Autodesk Inventor part; units mm, degrees
ref_plane "YZ Plane" through (0, 0, 0) normal (1, 0, 0) x (0, 1, 0)
ref_plane "XZ Plane" through (0, 0, 0) normal (0, 1, 0) x (-1, 0, 0)
ref_plane "XY Plane" through (0, 0, 0) normal (0, 0, 1) x (1, 0, 0)
sketch "Sketch1" plane through (0, 0, 0) normal (0, 1, 0) x (-1, 0, 0)
  line L0 (140, 140) -> (-140, 140)
  line L1 (-140, 140) -> (-140, -140)
  line L2 (-140, -140) -> (140, -140)
  line L3 (140, -140) -> (140, 140)
  point P0 (0, 0)
  point P1 (140, 0)
  point P2 (0, -140)
  dimension "d0" = 280
  dimension "d1" = 280
extrude "Extrusion1" add sketch "Sketch1" along normal blind 10
sketch "Sketch2" plane through (0, 10, 0) normal (0, 1, 0) x (1, 0, 0)
  line L0 (-140, -140) -> (140, -140)
  line L1 (140, -140) -> (140, 140)
  line L2 (140, 140) -> (-140, 140)
  line L3 (-140, 140) -> (-140, -140)
  line L4 (-132, -132) -> (132, -132)
  line L5 (132, -132) -> (132, 132)
  line L6 (132, 132) -> (-132, 132)
  line L7 (-132, 132) -> (-132, -132)
  point P0 (0, 0)
  dimension "d4" = 8
extrude "Extrusion2" add sketch "Sketch2" along normal blind 150
sketch "Sketch3" plane through (0, 160, 0) normal (0, 1, 0) x (1, 0, 0)
  circle A0 centre (-135, 135) radius 2.05
  circle A1 centre (135, 135) radius 2.05
  circle A2 centre (135, -135) radius 2.05
  circle A3 centre (-135, -135) radius 2.05
  line L0 (140, -140) -> (140, 140)
  line L1 (-140, -140) -> (140, -140)
  line L2 (140, 140) -> (-140, 140)
  line L3 (-140, 140) -> (-140, -140)
  point P0 (0, 0)
  dimension "d8" = 4.1
  dimension "d12" = 5
  dimension "d16" = 5
  dimension "d18" = 4.1
  dimension "d19" = 5
  dimension "d20" = 5
  dimension "d21" = 4.1
  dimension "d22" = 5
  dimension "d23" = 5
  dimension "d24" = 5
  dimension "d25" = 5
  dimension "d26" = 4.1
extrude "Extrusion3" cut sketch "Sketch3" against normal blind 15 contours A0 | A1 | A2 | A3
sketch "Sketch4" plane through (140, 0, 140) normal (1, 0, 0) x (0, 0, -1)
  line L0 (90, 130) -> (190, 130)
  line L1 (190, 130) -> (190, 30)
  line L2 (190, 30) -> (90, 30)
  line L3 (90, 30) -> (90, 130)
  line L4 (0, 160) -> (280, 160)
  line L5 (280, 0) -> (280, 160)
  point P0 (140, 0)
  point P1 (140, 130)
  point P2 (140, 160)
  point P3 (190, 80)
  point P4 (280, 80)
  dimension "d29" = 100
  dimension "d30" = 100
sketch "Sketch5" plane through (-140, 0, 140) normal (0, 0, 1) x (1, 0, 0)
  line L0 (280, 0) -> (280, 160)
  line L1 (0, 160) -> (280, 160)
  circle A0 centre (140, 80) radius 40.5
  point P0 (140, 0)
  point P1 (195.958, 80)
  point P2 (280, 80)
  point P3 (140, 107.0458)
  point P4 (140, 160)
  point P5 (280, 80)
  point P6 (140, 160)
  dimension "d81" = 81
extrude "Extrusion4" cut sketch "Sketch5" against normal blind 10
sketch "Sketch6" plane through (-140, 0, 140) normal (0, 0, 1) x (1, 0, 0)
  line L0 (192.5, 27.5) -> (87.5, 27.5)
  line L1 (87.5, 27.5) -> (87.5, 132.5)
  line L2 (87.5, 132.5) -> (192.5, 132.5)
  line L3 (192.5, 132.5) -> (192.5, 27.5)
  line L4 (0, 0) -> (280, 0)
  line L5 (0, 0) -> (0, 160)
  circle A0 centre (182.5, 37.5) radius 2.75
  circle A1 centre (182.5, 122.5) radius 2.75
  circle A2 centre (97.5, 37.5) radius 2.75
  circle A3 centre (97.5, 122.5) radius 2.75
  line L6 (210, 30) -> (70, 30)
  point P0 (140, 0)
  point P1 (49.5, 158)
  point P2 (180.5, 27)
  point P3 (140, 27.5)
  point P4 (140, 0)
  point P5 (87.5, 80)
  point P6 (0, 80)
  point P7 (60, 80)
  point P8 (140, 30)
  dimension "d108" = 105
  dimension "d109" = 105
  dimension "d112" = 5.5
  dimension "d113" = 10
  dimension "d114" = 10
  dimension "d117" = 85
  dimension "d120" = 85
sketch "Sketch7" plane through (0, 10, 0) normal (0, 1, 0) x (1, 0, 0)
  line L0 (132, 132) -> (132, -132) construction
  line L1 (132, 0) -> (-132, 0) construction
  line L2 (-132, -132) -> (-132, 132) construction
  point P0 (0, 0)
ref_plane "Work Plane1" through (132, 10, 0) normal (0, 0, -1) x (-1, 0, 0)
extrude "Extrusion13" cut sketch "Sketch6" against normal blind 5
mirror "Mirror2" about plane through (132, 10, 0) normal (0, 0, -1) of "Extrusion4"
sketch "Sketch8" plane through (0, 0, 0) normal (0, -1, 0) x (1, 0, 0)
  line L0 (75, -75) -> (-75, -75)
  line L1 (-75, -75) -> (-75, 75)
  line L2 (-75, 75) -> (75, 75)
  line L3 (75, 75) -> (75, -75)
  circle A0 centre (65, -65) radius 2.75
  circle A1 centre (65, 65) radius 2.75
  circle A2 centre (-65, -65) radius 2.75
  circle A3 centre (-65, 65) radius 2.75
  circle A4 centre (0, 0) radius 40.5
  point P0 (-35, 0)
  point P1 (0, -35)
  point P2 (75, 0)
  point P3 (0, -75)
  dimension "d58" = 130
  dimension "d65" = 130
  dimension "d82" = 81
  dimension "d83" = 150
  dimension "d84" = 150
  dimension "d85" = 10
  dimension "d86" = 10
  dimension "d87" = 130
  dimension "d88" = 130
  dimension "d89" = 5.5
  dimension "d90" = 5.5
  dimension "d91" = 5.5
  dimension "d92" = 5.5
extrude "Extrusion9" cut sketch "Sketch8" against normal blind 10 contours A4
sketch "Sketch13" plane through (0, 0, 0) normal (0, -1, 0) x (1, 0, 0)
  line L0 (-52.5, 52.5) -> (52.5, 52.5)
  line L1 (52.5, 52.5) -> (52.5, -52.5)
  line L2 (52.5, -52.5) -> (-52.5, -52.5)
  line L3 (-52.5, -52.5) -> (-52.5, 52.5)
  circle A0 centre (-42.5, 42.5) radius 2.75
  circle A1 centre (-42.5, -42.5) radius 2.75
  circle A2 centre (42.5, -42.5) radius 2.75
  circle A3 centre (42.5, 42.5) radius 2.75
  point P0 (0, 0)
  point P1 (52.5, 0)
  point P2 (0, 52.5)
  dimension "d95" = 105
  dimension "d96" = 105
  dimension "d97" = 5.5
  dimension "d98" = 10
  dimension "d99" = 10
  dimension "d102" = 360
extrude "Extrusion10" cut sketch "Sketch13" against normal blind 5
sketch "Sketch14" plane through (42.5, 0, 42.5) normal (0, -1, 0) x (1, 0, 0)
  circle A0 centre (0, 0) radius 2.75
  circle A1 centre (0, 0) radius 2.75
  circle A2 centre (0, -85) radius 2.75
  circle A3 centre (0, -85) radius 2.75
  circle A4 centre (-85, -85) radius 2.75
  circle A5 centre (-85, -85) radius 2.75
  circle A6 centre (-85, 0) radius 2.75
  circle A7 centre (-85, 0) radius 2.75
  point P0 (-42.5, -42.5)
extrude "Extrusion11" cut sketch "Sketch14" against normal up to next
sketch "Sketch16" plane through (-42.5, 122.5, 140) normal (0, 0, 1) x (1, 0, 0)
  circle A0 centre (0, 0) radius 2.75
  circle A1 centre (85, 0) radius 2.75
  circle A2 centre (85, 0) radius 2.75
  circle A3 centre (85, -85) radius 2.75
  circle A4 centre (85, -85) radius 2.75
  circle A5 centre (0, -85) radius 2.75
  circle A6 centre (0, -85) radius 2.75
  circle A7 centre (0, 0) radius 2.75
  point P0 (42.5, -122.5)
  dimension "d129" = 5.5
  dimension "d130" = 5.5
  dimension "d131" = 5.5
  dimension "d132" = 5.5
extrude "Extrusion14" cut sketch "Sketch16" against normal blind 10
mirror "Mirror4" about plane through (132, 10, 0) normal (0, 0, -1) of "Extrusion13", "Extrusion14"
properties part number "brain box bottom"
Part model, mm, in its own coordinate system. A direction names the side the tool comes from. Round coordinates to 2 decimals unless told otherwise and drop trailing zeros. Write each loop counter-clockwise with the first axis right and the second up, starting at its lowest first coordinate (ties: lowest second). Pieces come first, ordered by that corner, then holes. Notation, with made-up numbers: (47, 13.25) - (55, 13.25) arc R19 cw to (55, 42.25) - close; hole circle Ø8 at (-12.75, -22.75). An arc over 180 degrees is marked (long way). Use CSV: the item, a comma, the result in double quotes.
Item 1: Slice it at D-D, the plane z = 102. Write the cut outline in (x, y), then the cut area to 3 significant figures.
Results list:
outline,"(-140, 0) - (140, 0) - (140, 160) - (132, 160) - (132, 10) - (-132, 10) - (-132, 160) - (-140, 160) - close"
area,"5,200 mm²"
Item 2: Slice it at A-A, the plane z = 0. Write the cut outline in (x, y), then the cut area to 3 significant figures.
Results list:
outline,"(-140, 0) - (-52.5, 0) - (-52.5, 5) - (-40.5, 5) - (-40.5, 10) - (-132, 10) - (-132, 160) - (-140, 160) - close; (40.5, 5) - (52.5, 5) - (52.5, 0) - (140, 0) - (140, 160) - (132, 160) - (132, 10) - (40.5, 10) - close"
area,"4,270 mm²"
Item 3: Pull direction Y, two halves, no side cores. Call faces 1 (the flat face through (-1, 160, -135)), 2 (the cylindrical face through (-5.272, 39.845, -133.521)), 3 (the flat face through (-132, 84, -2)), 4 (the flat face through (-36, 104, 135)): pulls with the +Y half, pulls with the -Y half, needs draft (parallel to the pull), parting line crosses it, or undercut.
Results list:
face 1,"pulls with the +Y half"
face 2,"undercut"
face 3,"needs draft"
face 4,"undercut"
Item 4: Slice it at C-C, the plane x = 0. Count the separate pieces of the cut face and the enclosed holes in it, then the cut area to 3 significant figures.
Results list:
separate pieces,"4"
enclosed holes,"0"
area,"2,730 mm²"
Item 5: Wall check: L1, parallel to Z at x = 135, y = 149.5; L2, parallel to Y at x = -42.5, z = 132.8. Give the ranges that are in metal, low to high.
Results list:
L1,"z = -140 to -137.05, -132.95 to 132.95, 137.05 to 140"
L2,"y = 0 to 34.75, 40.25 to 119.75, 125.25 to 160"
Item 6: Tool access for faces 5 (the flat face through (132, 84, 2)), 6 (the flat face through (24, 116, -135)), 7 (the flat face through (-36, 5, 24)): list every direction of +Z, -Z, +X, -X, +Y, -Y with a clear straight run to the whole face (end or side of a thin tool).
Results list:
face 5,"+Y"
face 6,"-Z"
face 7,"-Y"
Item 7: Slice it at B-B, the plane y = 80. Write the cut outline in (x, z), then the cut area to 3 significant figures.
Results list:
outline,"(-140, -140) - (-52.5, -140) - (-52.5, -135) - (-40.5, -135) - (-40.5, -132) - (-132, -132) - (-132, 132) - (-40.5, 132) - (-40.5, 135) - (-52.5, 135) - (-52.5, 140) - (-140, 140) - close; (40.5, -135) - (52.5, -135) - (52.5, -140) - (140, -140) - (140, 140) - (52.5, 140) - (52.5, 135) - (40.5, 135) - (40.5, 132) - (132, 132) - (132, -132) - (40.5, -132) - close"
area,"7,170 mm²"
Item 8: Flat gauge pins, fed straight in: P1, Ø1.5, axis at x = -12, z = -82.5, coming from the +Y side; P2, Ø2, axis at x = 135, z = 136, coming from the +Y side. Where does each tip first touch, or does it go through?
Results list:
P1,"stops at y = 10"
P2,"stops at y = 145"
